Source: three-view drawing plus pictorial views. Frame: mm from the lowest corner of the part. Give positions to 0.01 mm unless a question says otherwise; leave off trailing zeros. Loops run counter-clockwise (first coordinate to the right, second up) from the corner with the lowest first, then second, coordinate; pieces in that order, holes last. Notation, with made-up numbers: M 1,80 L 21,80 A22 ccw 21,116 Z; hole C -21.75,85 d1. An arc over 180 degrees is marked long. Answer as a JSON object with one key per item and string values. Group by question number.
1) Ray query, L1, parallel to X at y = 6.5, z = 1.5; L2, parallel to Y at x = 10, z = 1.5; L3, parallel to Y at x = 2, z = 0.2. Return the intervals inside material, ascending.
2) Section query B-B on z = 1.1. Return loops of the section in (x, y).
3) Section query A-A on y = 7. Return loops of the section in (x, z).
4) First-contact query: P1, Ø0.5, axis at x = 4.5, z = 1.5, coming from the -Y side. Flat tip, straight axial feed; report the tip coordinate or a pass-through.
5) Section query C-C on x = 34. Return loops of the section in (y, z), plus the area to 3 significant figures.
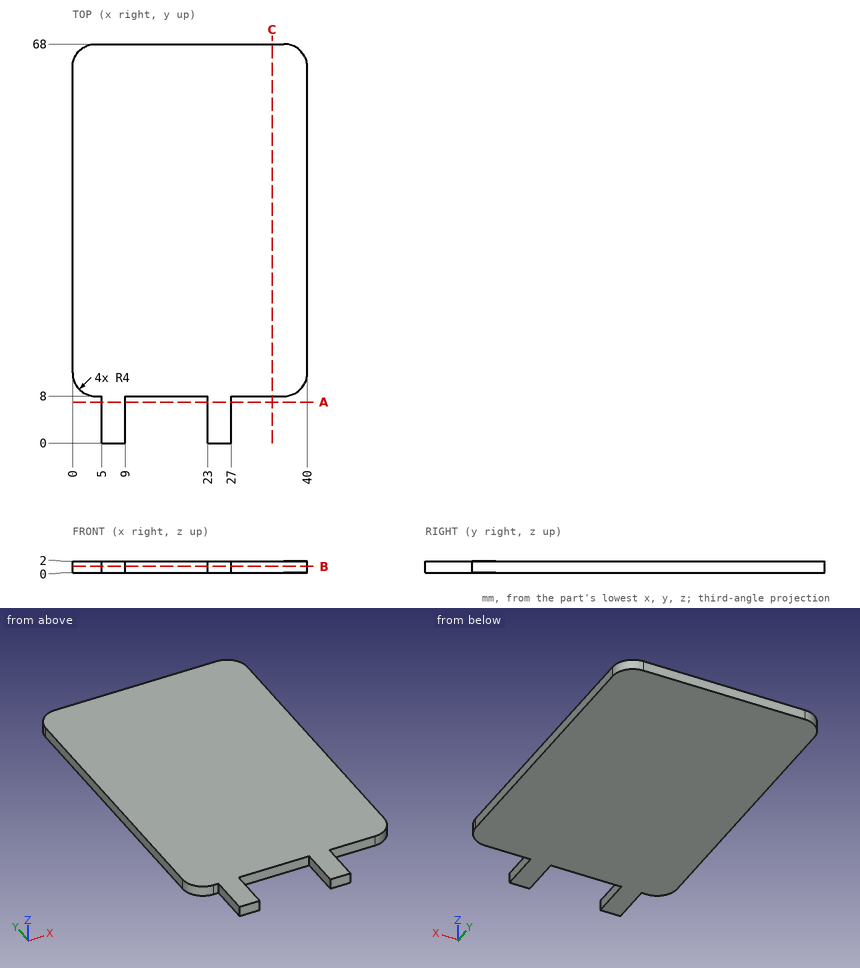
Output:
{
 "1": {"L1": "x = 5 to 9, 23 to 27", "L2": "y = 8 to 68", "L3": "y = 8.54 to 67.46"},
 "2": {"outline": "M 0,12 A4 ccw 4,8 L 5,8 L 5,0 L 9,0 L 9,8 L 23,8 L 23,0 L 27,0 L 27,8 L 36,8 A4 ccw 40,12 L 40,64 A4 ccw 36,68 L 4,68 A4 ccw 0,64 Z"},
 "3": {"outline": "M 5,0 L 9,0 L 9,2 L 5,2 Z; M 23,0 L 27,0 L 27,2 L 23,2 Z"},
 "4": {"P1": "stops at y = 8"},
 "5": {"outline": "M 8,0 L 68,0 L 68,2 L 8,2 Z", "area": "120 mm^2"}
}
